Print and shaded views of the part. All mm, measured from the part's lowest x, y and z. A direction names the side the tool comes from. Round coordinates to 2 decimals unless told otherwise and drop trailing zeros. Loops run counter-clockwise (first coordinate to the right, second up) from the corner with the lowest first, then second, coordinate; pieces in that order, holes last. Notation, with made-up numbers: (13.5, 21.5) - (28.5, 21.5) arc R17 ccw to (28.5, 33.5) - close; hole circle Ø4 at (87, 46.5). An arc over 180 degrees is marked (long way). Use one line per item in the form item = value.
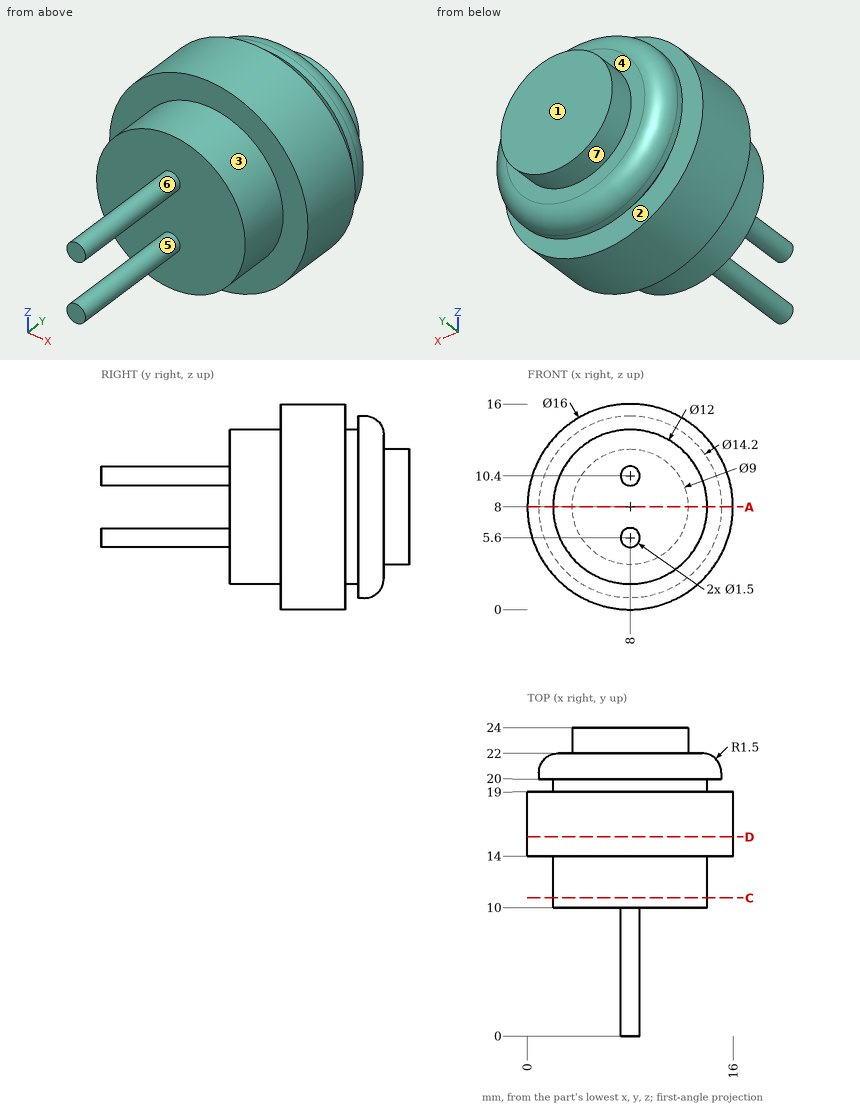
1. Cut at D-D, the plane y = 15.5. Give the cut face in (x, z).
Geometry check:
outline = circle Ø16 at (8, 8)
2. Cut at A-A, the plane z = 8. Give the cut face in (x, y).
Geometry check:
outline = (0, 14) - (2, 14) - (2, 10) - (14, 10) - (14, 14) - (16, 14) - (16, 19) - (14, 19) - (14, 20) - (15.1, 20) - (15.1, 20.5) arc R1.5 ccw to (13.6, 22) - (12.5, 22) - (12.5, 24) - (3.5, 24) - (3.5, 22) - (2.4, 22) arc R1.5 ccw to (0.9, 20.5) - (0.9, 20) - (2, 20) - (2, 19) - (0, 19) - close
3. Wall check: probe 1 along Z at (x, y) = (7.75, 14.75); probe 2 along Y at (x, z) = (9.5, 14.5); probe 3 along Y at (x, z) = (5, 8.25). Give the ranges that are in metal, low to high.
Geometry check:
probe_1 = 0 to 16
probe_2 = 14 to 19, 20 to 21.55
probe_3 = 10 to 24
4. Tool access for the marked faces 1, 2 and 3: list every direction of +Z, -Z, +X, -X, +Y, -Y with a clear straight run to the whole face (end or side of a thin tool).
Geometry check:
face_1 = +Z, -Z, +X, -X, +Y
face_2 = none
face_3 = -Y
5. Cut at C-C, the plane y = 10.75. Give the cut face in (x, z), plus the area to 3 significant figures.
Geometry check:
outline = circle Ø12 at (8, 8)
area = 113 mm^2
6. Flat gauge pins, fed straight in: pin 1 (3 mm diameter, centred on y = 18.5, z = 13, fed in from -X); pin 2 (2 mm diameter, centred on y = 4, z = 4.5, fed in from -X); pin 3 (2 mm diameter, centred on y = 20.5, z = 10, fed in from -X). Where does each tip first touch, or does it go through?
Geometry check:
pin_1 = 0.81
pin_2 = 7.26
pin_3 = 0.97
7. Pull direction Z, two halves, no side cores. Call the marked faces 4, 5, 6 and 7: +Z half, -Z half, draft (parallel to the pull), parting line (faces both ways), or undercut.
Geometry check:
face_4 = draft
face_5 = undercut
face_6 = undercut
face_7 = parting line
